Can you work these out from the model? Positions are in its coordinate system, mm. A direction names the side the tool comes from. Give positions to 0.01 mm unless a question says otherwise; leave off trailing zeros. Write each loop counter-clockwise with the first axis right and the second up, starting at its lowest first coordinate (ties: lowest second). Pieces come first, ordered by that corner, then holes. Notation, with made-up numbers: (77, 23) -> (81, 23) arc R20 cw to (81, 52) -> close; hole circle Ø6 at (32, 43.5). An arc over 180 degrees is marked (long way). Answer as CSV lines item,"result". Start each with the question number.
1. I need wall thicknesses on line 1 (Y direction, x = 10, z = 4.25); line 2 (X direction, y = 11.5, z = 3.5); line 3 (Y direction, x = 28, z = -1). Which ranges of each line are inside material? Lowest first, please. Write a range as [from, to].
2. If we section it at D-D on x = 10: Write out the boundary of the cut face in (y, z), plus the area to 3 significant figures.
3. If we section it at A-A on x = -5: Write out the boundary of the cut face in (y, z).
4. If we mould it in two halves opening along X, with no side actions, what happens to faces 6 (the face through (-35.835, 17.625, 4.93)), 7 (the face through (28.017, 20.518, -10.229)), 8 (the face through (20, 0, 2))? For each: pulls with the +X half, pulls with the -X half, needs draft (parallel to the pull), parting line crosses it, or undercut.
5. I'm going to push flat-ended pins straight in: P1, Ø5, axis at y = 8.5, z = -18, coming from the -X side; P2, Ø3, axis at y = -7.06, z = -17.95, coming from the +X side; P3, Ø6, axis at y = -3.5, z = -13, coming from the -X side; P4, Ø6, axis at y = 7.94, z = -1.95, coming from the -X side. Where does each tip first touch, or does it pass through?
6. If we section it at C-C on z = -17.95: Write out the boundary of the cut face in (x, y), plus the area to 3 significant figures.
7. On a 3-axis mill with a long thin cutter (end or side, diameter ignored), from which of +Z, -Z, +X, -X, +Y, -Y can I reach the whole of each face in a straight line? I mean faces 1 (the face through (-20, 0, 0)), 2 (the face through (29.2, 6.16, -18.18)), 3 (the face through (25.188, -7.198, -21.197)), 4 (the face through (26.864, -5.66, -0.55)), 5 (the face through (17.45, -19.04, 0.99)). Say none if no direction works.
8. If we section it at B-B on y = 3: Write out the boundary of the cut face in (x, z), plus the area to 3 significant figures.
Autodesk Inventor part; units mm, degrees
ref_plane "YZ Plane" through (0, 0, 0) normal (1, 0, 0) x (0, 1, 0)
ref_plane "XZ Plane" through (0, 0, 0) normal (0, 1, 0) x (-1, 0, 0)
ref_plane "XY Plane" through (0, 0, 0) normal (0, 0, 1) x (1, 0, 0)
sketch "Sketch1" plane through (0, 0, 0) normal (0, 0, 1) x (1, 0, 0)
  arc A0 (18.1843, -16.5324) -> (18.7618, -13.101) centre (16.0629, -14.4111) ccw
  arc A1 (18.7618, 13.101) -> (18.7618, -13.101) centre (45.75, 0) ccw
  arc A2 (18.7618, 13.101) -> (18.1843, 16.5324) centre (16.0629, 14.4111) ccw
  line L0 (11.5324, 23.1843) -> (18.1843, 16.5324)
  arc A3 (11.5324, 23.1843) -> (8.101, 23.7618) centre (9.4111, 21.0629) ccw
  arc A4 (-18.101, 23.7618) -> (8.101, 23.7618) centre (-5, 50.75) ccw
  arc A5 (-18.101, 23.7618) -> (-21.5324, 23.1843) centre (-19.4111, 21.0629) ccw
  line L1 (-28.1843, 16.5324) -> (-21.5324, 23.1843)
  arc A6 (-28.1843, 16.5324) -> (-28.7618, 13.101) centre (-26.0629, 14.4111) ccw
  arc A7 (-28.7618, -13.101) -> (-28.7618, 13.101) centre (-55.75, 0) ccw
  arc A8 (-28.7618, -13.101) -> (-28.1843, -16.5324) centre (-26.0629, -14.4111) ccw
  line L2 (-21.5324, -23.1843) -> (-28.1843, -16.5324)
  arc A9 (-21.5324, -23.1843) -> (-18.101, -23.7618) centre (-19.4111, -21.0629) ccw
  arc A10 (8.101, -23.7618) -> (-18.101, -23.7618) centre (-5, -50.75) ccw
  arc A11 (8.101, -23.7618) -> (11.5324, -23.1843) centre (9.4111, -21.0629) ccw
  line L3 (18.1843, -16.5324) -> (11.5324, -23.1843)
  circle A12 centre (10, -15) radius 4
  circle A13 centre (-20, -15) radius 4
  circle A14 centre (-20, 15) radius 4
  circle A15 centre (10, 15) radius 4
  circle A16 centre (-5, 0) radius 13
  line L4 (39.4645, -4.5) -> (34.9645, -4.5)
  line L5 (34.9645, -4.5) -> (34.9645, 4.5)
  line L6 (34.9645, 4.5) -> (39.4645, 4.5)
  line L7 (39.4645, 4.5) -> (39.4645, 10)
  line L8 (39.4645, 10) -> (31.4645, 10)
  line L9 (31.4645, 10) -> (31.4645, -10)
  line L10 (31.4645, -10) -> (39.4645, -10)
  line L11 (39.4645, -10) -> (39.4645, -4.5)
  line L12 (31.4645, -10) -> (31.4645, -17.0711)
  line L13 (31.4645, -17.0711) -> (24.4726, -24.0629)
  line L14 (31.4645, 10) -> (31.4645, 17.0711)
  line L15 (-19.4111, -24.0629) -> (24.4726, -24.0629)
  line L16 (-19.4111, 24.0629) -> (24.4726, 24.0629)
  line L17 (31.4645, 17.0711) -> (24.4726, 24.0629)
  circle A17 centre (-46, 0) radius 12.5
  line L18 (-20.5407, -23.8421) -> (-50.7071, -11.5799)
  line L19 (-50.7071, 11.5799) -> (-20.5407, 23.8421)
  point P0 (0, 0)
  dimension "d0" = 45
  dimension "d1" = 5
  dimension "d4" = 46
  dimension "d5" = 25
extrude "Extrusion1" add sketch "Sketch1" along normal blind 10 contours L3 A11 A10 A9 L2 A8 A7 A6 L1 A5 A4 A3 L0 A2 A1 A0 | A0 A1 A2 L0 A3 L16 L17 L14 L9 L12 L13 L15 A11 L3 | L15 A9 A10 A11 | L18 A17 L19 A5 L1 A6 A7 A8 L2 A9 | A3 A4 A5 L16 | A17
sketch "Sketch2" plane through (0, 0, 0) normal (0, 0, -1) x (-1, 0, 0)
  line L0 (-24.4726, -24.0629) -> (-31.4645, -17.0711)
  line L1 (19.4111, -24.0629) -> (-24.4726, -24.0629)
  arc A0 (19.4111, -24.0629) -> (20.5407, -23.8421) centre (19.4111, -21.0629) ccw
  line L2 (50.7071, -11.5799) -> (20.5407, -23.8421)
  arc A1 (50.7071, -11.5799) -> (50.7071, 11.5799) centre (46, 0) ccw
  line L3 (20.5407, 23.8421) -> (50.7071, 11.5799)
  arc A2 (20.5407, 23.8421) -> (19.4111, 24.0629) centre (19.4111, 21.0629) ccw
  line L4 (-24.4726, 24.0629) -> (19.4111, 24.0629)
  line L5 (-31.4645, 17.0711) -> (-24.4726, 24.0629)
  line L6 (-31.4645, -17.0711) -> (-31.4645, 17.0711)
  circle A3 centre (-10, -15) radius 4
  circle A4 centre (20, -15) radius 4
  circle A5 centre (20, 15) radius 4
  circle A6 centre (-10, 15) radius 4
  circle A7 centre (5, 0) radius 13
  line L7 (-31.4645, 17.0711) -> (-23.4645, 17.0711)
  line L8 (-23.4645, 17.0711) -> (-23.4645, -17.0711)
  line L9 (-24.4726, -24.0629) -> (-31.4645, -17.0711)
  line L10 (-23.4645, -17.0711) -> (-31.4645, -17.0711)
  line L11 (-23.4645, 17.0711) -> (-19.4726, 21.0629)
  line L12 (-19.4726, 21.0629) -> (-19.4726, 24.0629)
  line L13 (-23.4645, -17.0711) -> (-19.4726, -21.0629)
  line L14 (-19.4726, -21.0629) -> (-19.4726, -24.0629)
  line L15 (19.4111, -24.0629) -> (-24.4726, -24.0629)
  point P0 (0, 0)
  dimension "d6" = 8
  dimension "d9" = 3
extrude "Extrusion2" add sketch "Sketch2" along normal blind 29.9 contours L0 L10 L13 L14 L1 | L6 L7 L8 L10 | L5 L4 L12 L11 L7
sketch "Sketch3" plane through (23.4645, -17.0711, 0) normal (-1, 0, 0) x (0, 0, 1)
  line L0 (0, 34.1421) -> (0, 0)
  line L1 (0, 34.1421) -> (-29.9, 34.1421)
  line L2 (-29.9, 0) -> (-29.9, 34.1421)
  line L3 (0, 0) -> (-29.9, 0)
  point P0 (0, 17.0711)
  point P1 (-1.95, 25.0158)
  point P2 (-17.95, 25.0158)
  point P3 (-17.95, 10.0158)
  point P4 (-1.95, 10.0158)
  dimension "d10" = 15
  dimension "d11" = 16
  dimension "d12" = 11.95
hole "Hole1" at (23.4645, 7.9447, -1.95) at (23.4645, 7.9447, -17.95) at (23.4645, -7.0553, -17.95) at (23.4645, -7.0553, -1.95) direction (1, 0, 0) diameter 3.6 end through all counterbore diameter 6.5 counterbore depth 3.4
sketch "Sketch4" plane through (0, 0, 0) normal (0, 0, -1) x (-1, 0, 0)
  circle A0 centre (5, 0) radius 13
  circle A1 centre (-10, 15) radius 4
  circle A2 centre (20, 15) radius 4
  circle A3 centre (20, -15) radius 4
  circle A4 centre (-10, -15) radius 4
  line L0 (-19.4726, 24.0629) -> (-19.4726, 21.0629)
  line L1 (-19.4726, 21.0629) -> (-23.4645, 17.0711)
  line L2 (-23.4645, 17.0711) -> (-23.4645, 10.5447)
  line L3 (-23.4645, 10.5447) -> (-23.4645, 5.3447)
  line L4 (-23.4645, 5.3447) -> (-23.4645, -4.4553)
  line L5 (-23.4645, -4.4553) -> (-23.4645, -9.6553)
  line L6 (-23.4645, -9.6553) -> (-23.4645, -17.0711)
  line L7 (-23.4645, -17.0711) -> (-19.4726, -21.0629)
  line L8 (-19.4726, -21.0629) -> (-19.4726, -24.0629)
  line L9 (19.4111, -24.0629) -> (-19.4726, -24.0629)
  arc A5 (19.4111, -24.0629) -> (20.5407, -23.8421) centre (19.4111, -21.0629) ccw
  line L10 (50.7071, -11.5799) -> (20.5407, -23.8421)
  arc A6 (50.7071, -11.5799) -> (50.7071, 11.5799) centre (46, 0) ccw
  line L11 (20.5407, 23.8421) -> (50.7071, 11.5799)
  arc A7 (20.5407, 23.8421) -> (19.4111, 24.0629) centre (19.4111, 21.0629) ccw
  line L12 (-19.4726, 24.0629) -> (19.4111, 24.0629)
  line L13 (-19.4726, 21.0629) -> (-15.4807, 17.0711)
  line L14 (-15.4807, 17.0711) -> (-15.4807, -17.0711)
  line L15 (-15.4807, -17.0711) -> (-19.4726, -21.0629)
  line L16 (-23.4645, 17.0711) -> (-19.4726, 21.0629)
  point P0 (0, 0)
extrude "Extrusion3" cut sketch "Sketch4" against normal blind 2 contours L13 L14 L15 L7 L6 L5 L4 L3 L2 L1
properties part number "Rear Z Axis Carriage" material "ABS Plastic"
Computed values:
1,line 1,"y = [-24.06, -19], [-11, 11], [19, 24.06]"
1,line 2,"x = [-50.9, -21.94], [-18.06, -11.06], [1.06, 8.06], [11.94, 31.46]"
1,line 3,"y = [-20.54, -8.58], [-5.53, 6.42], [9.47, 20.54]"
2,outline,"(-24.06, 0) -> (-19, 0) -> (-19, 10) -> (-24.06, 10) -> close; (-11, 0) -> (11, 0) -> (11, 10) -> (-11, 10) -> close; (19, 0) -> (24.06, 0) -> (24.06, 10) -> (19, 10) -> close"
2,area,"321 mm2"
3,outline,"(-24.06, 0) -> (-13, 0) -> (-13, 10) -> (-24.06, 10) -> close; (13, 0) -> (24.06, 0) -> (24.06, 10) -> (13, 10) -> close"
4,face 6,"pulls with the -X half"
4,face 7,"pulls with the +X half"
4,face 8,"undercut"
5,P1,"stops at x = 26.86"
5,P2,"passes through"
5,P3,"stops at x = 23.46"
5,P4,"stops at x = -57.15"
6,outline,"(19.47, -24.06) -> (24.47, -24.06) -> (31.46, -17.07) -> (31.46, -8.86) -> (26.86, -8.86) -> (26.86, -10.31) -> (23.46, -10.31) -> (23.46, -17.07) -> (19.47, -21.06) -> close; (19.47, 21.06) -> (23.46, 17.07) -> (23.46, 11.19) -> (26.86, 11.19) -> (26.86, 9.74) -> (31.46, 9.74) -> (31.46, 17.07) -> (24.47, 24.06) -> (19.47, 24.06) -> close; (23.46, -3.81) -> (26.86, -3.81) -> (26.86, -5.26) -> (31.46, -5.26) -> (31.46, 6.14) -> (26.86, 6.14) -> (26.86, 4.69) -> (23.46, 4.69) -> close"
6,area,"299 mm2"
7,face 1,"-Z, -X, +Y, -Y"
7,face 2,"+X, -X"
7,face 3,"-X"
7,face 4,"none"
7,face 5,"-Z"
8,outline,"(-58.13, 0) -> (-17.65, 0) -> (-17.65, 10) -> (-58.13, 10) -> close; (7.65, 0) -> (15.48, 0) -> (15.48, 2) -> (23.46, 2) -> (23.46, -29.9) -> (31.46, -29.9) -> (31.46, 10) -> (7.65, 10) -> close"
8,area,"866 mm2"
